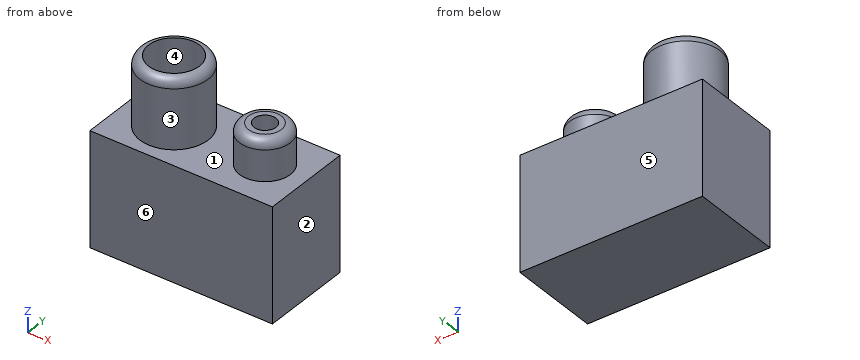
from build123d import *

# Parameters (mm, degrees)
F0_W     = 101.6528531909
F0_H     = 50.9243570268
F1_DEPTH = 63.5
F2_R     = 19.0350145172
F3_DEPTH = 38.1
F4_R     = 14.1510097993
F5_DEPTH = 38.1
F6_W     = 8.0858180299
F6_H     = 29.7073572874


# Not quite as in the source:
# - a fillet or chamfer that OpenCascade refuses, or shapes differently, is made with other operations: its cross-section is extruded or revolved along the edge and cut away or added


with BuildPart() as f1:
    # F0 (on Top) → F1 (new body)
    with BuildSketch(Plane.XY):
        Rectangle(F0_W, F0_H)
    extrude(amount=F1_DEPTH)

    # F2 (on face) → F3 (join)
    with BuildSketch(Plane.XY.offset(63.5)):
        with Locations((-22.8180289268, 0)):
            Circle(F2_R)
    extrude(amount=F3_DEPTH)

    # F4 (on face) → F5 (cut, through all)
    with BuildSketch(Plane.XY.offset(101.6)):
        with Locations((-22.8180289268, 0)):
            Circle(F4_R)
    extrude(amount=-F5_DEPTH, mode=Mode.SUBTRACT)

    # F6 (on Front) → F7 (revolve)
    with BuildSketch(Plane.XZ):
        with Locations((17.6577321254, 70.9035620093)):
            Rectangle(F6_W, F6_H)
    revolve(axis=Axis((27.8174318373, 0, 58.8010009378), (0, 0, -1)))

    # F8: fillet of radius 5.08 on 2 edges, made by hand

    # F8_s1 → F8_t2 (revolve, cut)
    with BuildSketch(Plane.XZ):
        with BuildLine():
            ThreePointArc((-3.7830144096, 96.5237823284), (-5.2022729524, 100.0459083885), (-8.6670191276, 101.6))
            Line((-8.6670191276, 101.6), (-3.7830144096, 101.6))
            Line((-3.7830144096, 101.6), (-3.7830144096, 96.5237823284))
        make_face()
    revolve(axis=Axis((-22.8180289268, 0, 101.6), (0, 0, 1)), mode=Mode.SUBTRACT)

    # F8_s3 → F8_t4 (revolve, cut)
    with BuildSketch(Plane.XZ):
        with BuildLine():
            ThreePointArc((13.6148231104, 80.677240653), (15.102720662, 84.2693431015), (18.6948231104, 85.757240653))
            Line((18.6948231104, 85.757240653), (13.6148231104, 85.757240653))
            Line((13.6148231104, 85.757240653), (13.6148231104, 80.677240653))
        make_face()
    revolve(axis=Axis((27.8174318373, 0, 85.757240653), (0, 0, -1)), mode=Mode.SUBTRACT)


solid = f1.part
Work out the finished part from the listing and answer in its coordinate system (mm). Face numbers are marked on the shaded views. A direction names the side the tool comes from. Round coordinates to 2 decimals unless told otherwise and drop trailing zeros. Write each loop counter-clockwise with the first axis right and the second up, starting at its lowest first coordinate (ties: lowest second). Pieces come first, ordered by that corner, then holes.
1) The mould has two halves that part along Y. Classify the marked faces 3, 4, 5 and 6: pulls with the +Y half, pulls with the -Y half, needs draft (parallel to the pull), parting line crosses it, or undercut.
2) A cutting plane is placed at C-C (z = 94.5). Give the vertices of the cut face in (x, y).
3) A cutting plane is placed at B-B (y = 0). Give the vertices of the cut face in (x, z), plus the area to 3 significant figures.
4) A cutting plane is placed at D-D (x = 10). Give the vertices of the cut face in (y, z), plus the area to 3 significant figures.
5) Given pin 1 Ø5 at (y, z) = (-9, 76.5) entering from +X; pin 2 Ø20 at (x, y) = (32, 4) entering from +Z; pin 3 Ø1.5 at (x, y) = (-11, 1) entering from +Z, each flat-ended and moving along its own axis, determine where each tip first touches the part or whether it passes through.
6) Straight lines are drawn through the part: line 1 (X direction, y = 12.5, z = 77.5); line 2 (Z direction, x = -45, y = 10.5); line 3 (Y direction, x = 27, z = 75). For each, find the intervals that lie inside material, in ascending order.
7) A tool of negligible diameter and unlimited length cuts with its end or side. For the marked faces 1 and 2, from which of +Z, -Z, +X, -X, +Y, -Y can it reach the whole face along a straight path? Write none if from no direction.
8) A cutting plane is placed at A-A (z = 74). Give the vertices of the cut face in (x, y).
Completed:
1. face 3: parting line crosses it
1. face 4: undercut
1. face 5: pulls with the +Y half
1. face 6: pulls with the -Y half
2. outline: circle Ø38.07 at (-22.82, 0); hole circle Ø28.3 at (-22.82, 0)
3. outline: (-50.83, 0) - (50.83, 0) - (50.83, 63.5) - (42.02, 63.5) - (42.02, 80.68) arc R5.08 ccw to (36.94, 85.76) - (33.93, 85.76) - (33.93, 63.5) - (21.7, 63.5) - (21.7, 85.76) - (18.69, 85.76) arc R5.08 ccw to (13.61, 80.68) - (13.61, 63.5) - (-3.78, 63.5) - (-3.78, 96.52) arc R5.08 ccw to (-8.67, 101.6) - (-8.67, 63.5) - (-36.97, 63.5) - (-36.97, 101.6) arc R5.08 ccw to (-41.85, 96.52) - (-41.85, 63.5) - (-50.83, 63.5) - close
3. area: 7,160 mm2
4. outline: (-25.46, 0) - (25.46, 0) - (25.46, 63.5) - (-25.46, 63.5) - close
4. area: 3,230 mm2
5. pin 1: stops at x = 40.45
5. pin 2: stops at z = 85.76
5. pin 3: stops at z = 63.5
6. line 1: x = -37.17 to -29.45, -16.18 to -8.46, 21.07 to 34.56
6. line 2: z = 0 to 63.5
6. line 3: y = -14.18 to -6.06, 6.06 to 14.18
7. face 1: +Z
7. face 2: +Z, -Z, +X, +Y, -Y
8. outline: circle Ø38.07 at (-22.82, 0); circle Ø28.41 at (27.82, 0); hole circle Ø28.3 at (-22.82, 0); hole circle Ø12.23 at (27.82, 0)
